Read the model definition and answer for the solid it produces. Units are mm, in the model's axes. A direction names the side the tool comes from. Give positions to 0.01 mm unless a question says otherwise; leave off trailing zeros. Write each loop counter-clockwise with the first axis right and the second up, starting at its lowest first coordinate (ties: lowest second). Pieces come first, ordered by that corner, then holes. Notation, with made-up numbers: M -36,16.5 L -3,16.5 A21 ccw -3,20.5 Z; hole C 63.25,-24 d6. An arc over 180 degrees is marked long. Answer as CSV lines item,"result". Start each with the question number.
```python
from build123d import *

# Parameters (mm, degrees)
F1_DEPTH = 50
F3_DEPTH = 10
F4_R     = 4
F5_DEPTH = 15


with BuildPart() as f1:
    # F0 (on Top) → F1 (new body)
    with BuildSketch(Plane.XY):
        Polygon((0, 92.5), (0, 0), (2.5, 0), (2.5, 90), (44.5, 90), (44.5, 35), (47, 35), (47, 92.5), align=None)
    extrude(amount=F1_DEPTH)

    # F2 (on face) → F3 (join)
    with BuildSketch(Plane.YZ.offset(2.5)):
        with BuildLine():
            Line((22.68132, 40.430217), (17.5, 41.689106))
            Line((17.5, 41.689106), (17.5, 39.416046))
            ThreePointArc((17.5, 39.416046), (20.622616, 38.122616), (21.916046, 35))
            ThreePointArc((21.916046, 35), (20.622616, 31.877384), (17.5, 30.583954))
            Line((17.5, 30.583954), (17.5, 28.310894))
            Line((17.5, 28.310894), (19.612045, 27.797737))
            Line((19.612045, 27.797737), (24.793366, 33.227953))
            Line((24.793366, 33.227953), (22.68132, 40.430217))
        make_face()
        with BuildLine():
            Line((17.5, 39.416046), (17.5, 41.689106))
            Line((17.5, 41.689106), (15.387955, 42.202263))
            Line((15.387955, 42.202263), (10.206634, 36.772047))
            Line((10.206634, 36.772047), (12.31868, 29.569783))
            Line((12.31868, 29.569783), (17.5, 28.310894))
            Line((17.5, 28.310894), (17.5, 30.583954))
            ThreePointArc((17.5, 30.583954), (13.083954, 35), (17.5, 39.416046))
        make_face()
        with BuildLine():
            ThreePointArc((21.304212, 15), (20.189984, 17.689984), (17.5, 18.804212))
            ThreePointArc((17.5, 18.804212), (14.810016, 12.310016), (21.304212, 15))
        make_face()
        Polygon((21.857131, 21.111362), (17.5, 21.529923), (14.385971, 21.829067), (10.02884, 15.717706), (13.142869, 8.888638), (20.614029, 8.170933), (24.97116, 14.282294), align=None)
        with BuildLine():
            ThreePointArc((21.304212, 15), (14.810016, 12.310016), (17.5, 18.804212))
            ThreePointArc((17.5, 18.804212), (20.189984, 17.689984), (21.304212, 15))
        make_face(mode=Mode.SUBTRACT)
    extrude(amount=-F3_DEPTH)

    # F4 (on face) → F5 (cut)
    with BuildSketch(Plane.YZ.offset(2.5)):
        with Locations((17.5, 35)):
            Circle(F4_R)
        with Locations((17.5, 15)):
            Circle(F4_R)
    extrude(amount=-F5_DEPTH, mode=Mode.SUBTRACT)


solid = f1.part
```
1. Find the intervals of material crossed by line 1 (Z direction, x = 0.6, y = 17.5); line 2 (X direction, y = 54, z = 19.5); line 3 (Y direction, x = 25.5, z = 23), in increasing order. Write a range as [from, to].
2. Find section B-B on z = 45.5. Determine the outline of the cut face in (x, y).
3. For faces 1 (the face through (-3.7, 11.25, 33.22)), 2 (the face through (46, 35, 25)), 3 (the face through (-3.698, 22.166, 30.475)), determine the directions among +Z, -Z, +X, -X, +Y, -Y from which every point of the face is accessible in a straight line to the end or side of a thin tool.
4. Find section A-A on y = 48. Determine the outline of the cut face in (x, z), then the cut area to 3 significant figures.
5. Find section D-D on x = 40.5. Determine the outline of the cut face in (y, z).
6. Determine the mould class of faces 4 (the face through (1, 67, 0)), 5 (the face through (23, 90, 25)), 6 (the face through (-7.5, 14, 38)) for opening direction X: +X half, -X half, draft (parallel to the pull), parting line (faces both ways), or undercut.
7. Given pin 1 (0.8 mm diameter, centred on x = 45.5, z = 22, fed in from -Y); pin 2 (2 mm diameter, centred on y = 63, z = 9.5, fed in from -X); pin 3 (5 mm diameter, centred on x = 22.5, z = 12, fed in from -Y), each flat-ended and moving along its own axis, determine where each tip first touches the part or whether it passes through.
8. Find section C-C on y = 16.5. Determine the outline of the cut face in (x, z), then the cut area to 3 significant figures.
Computed:
1,line 1,"z = [0, 11], [19, 31], [39, 50]"
1,line 2,"x = [0, 2.5], [44.5, 47]"
1,line 3,"y = [90, 92.5]"
2,outline,"M 0,0 L 2.5,0 L 2.5,90 L 44.5,90 L 44.5,35 L 47,35 L 47,92.5 L 0,92.5 Z"
3,face 1,"-X, -Y"
3,face 2,"+Z, -Z, +X, -Y"
3,face 3,"-X, +Y"
4,outline,"M 0,0 L 2.5,0 L 2.5,50 L 0,50 Z; M 44.5,0 L 47,0 L 47,50 L 44.5,50 Z"
4,area,"250 mm^2"
5,outline,"M 90,0 L 92.5,0 L 92.5,50 L 90,50 Z"
6,face 4,"draft"
6,face 5,"undercut"
6,face 6,"-X half"
7,pin 1,"stops at y = 35"
7,pin 2,"stops at x = 0"
7,pin 3,"stops at y = 90"
8,outline,"M -7.5,8.57 L 0,8.57 L 0,0 L 2.5,0 L 2.5,11.13 L -7.5,11.13 Z; M -7.5,18.87 L 2.5,18.87 L 2.5,31.13 L 0,31.13 L 0,30.7 L -7.5,30.7 L -7.5,28.55 L 0,28.55 L 0,21.63 L -7.5,21.63 Z; M -7.5,39.3 L 0,39.3 L 0,38.87 L 2.5,38.87 L 2.5,50 L 0,50 L 0,41.93 L -7.5,41.93 Z"
8,area,"162 mm^2"
